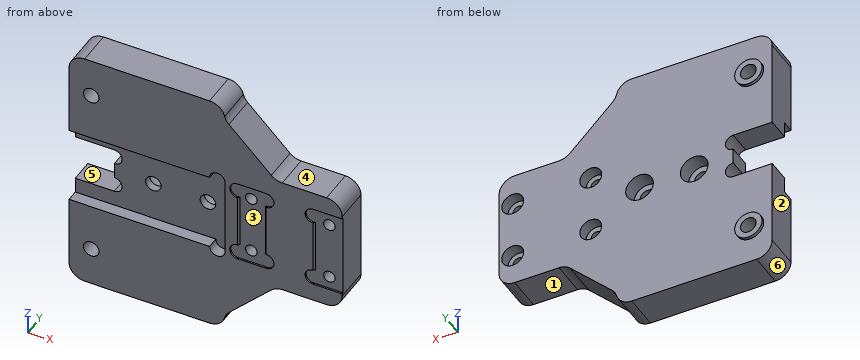
from build123d import *

# Parameters (mm, degrees)
SKETCH1_R               = 12
BOSS_EXTRUDE1_DEPTH     = 4.5
SKETCH2_R               = 1.7
CUT_EXTRUDE1_DEPTH      = 91.980767198
FILLET1_R               = 4
CUT_EXTRUDE4_DEPTH      = 91.980767198
FILLET3_R               = 4
SKETCH6_R               = 1.5
CUT_EXTRUDE5_DEPTH      = 41
CUT_EXTRUDE6_START      = -6
SKETCH7_W               = 30
SKETCH7_H               = 20
CUT_EXTRUDE6_DEPTH      = 3
SKETCH8_W               = 60
SKETCH8_H               = 17
CUT_EXTRUDE8_DEPTH      = 9
FILLET6_R               = 4
SKETCH9_W               = 40
SKETCH9_H               = 22.25
BOSS_EXTRUDE3_DEPTH     = 9
FILLET7_R               = 4
SKETCH13_R              = 3.5
BOSS_EXTRUDE5_DEPTH     = 0.8
CUT_EXTRUDE9_DEPTH      = 2
CUT_EXTRUDE9_DEPTH_BACK = 9
SKETCH10_R              = 2
BOSS_EXTRUDE4_DEPTH     = 9
SKETCH14_R              = 2
CUT_EXTRUDE10_DEPTH     = 16
SKETCH15_W              = 7.5
SKETCH15_H              = 21.7
CUT_EXTRUDE11_DEPTH     = 0.4
CHAMFER2_SIZE           = 0.4
CHAMFER3_SIZE           = 0.6
SKETCH16_W              = 4
SKETCH16_H              = 6
BOSS_EXTRUDE6_DEPTH     = 10
SKETCH17_R              = 2
CUT_EXTRUDE12_DEPTH     = 12.4
SKETCH18_R              = 3.55
CUT_EXTRUDE13_DEPTH     = 4
SKETCH19_R              = 2.8
CUT_EXTRUDE14_DEPTH     = 3
SKETCH20_R              = 2
CUT_EXTRUDE15_DEPTH     = 0.4
FILLET8_R               = 4
SKETCH21_R              = 2
CUT_EXTRUDE16_DEPTH     = 3


# Some blends are built 0.0001 mm under size
with BuildPart() as part:
    # Sketch1 → Boss-Extrude1 (new, symmetric)
    with BuildSketch(Plane(origin=(0, 0, 0), x_dir=(1, 0, 0), z_dir=(0, 1, 0))):
        Polygon((21.5, 20), (21.5, -20), (-20.5, -32.5), (-84.5, -32.5), (-84.5, 32.5), (-20.5, 32.5), align=None)
        with Locations(Location((0, 0, 0), (0, 0, 270))):
            Circle(SKETCH1_R, mode=Mode.SUBTRACT)
    extrude(amount=BOSS_EXTRUDE1_DEPTH, both=True)

    # Sketch2 → Cut-Extrude1 (cut, through all)
    with BuildSketch(Plane(origin=(0, 4.5, 0), x_dir=(1, 0, 0), z_dir=(0, 1, 0))):
        with Locations(Location((15.5, 15.5, 0), (0, 0, 270))):
            Circle(SKETCH2_R)
        with Locations(Location((-15.5, 15.5, 0), (0, 0, 270))):
            Circle(SKETCH2_R)
        with Locations(Location((-15.5, -15.5, 0), (0, 0, 270))):
            Circle(SKETCH2_R)
        with Locations(Location((15.5, -15.5, 0), (0, 0, 270))):
            Circle(SKETCH2_R)
        with Locations(Location((-19.5, 27.5, 0), (0, 0, 270))):
            Circle(SKETCH2_R)
        with Locations(Location((-19.5, -27.5, 0), (0, 0, 270))):
            Circle(SKETCH2_R)
    extrude(amount=-CUT_EXTRUDE1_DEPTH, mode=Mode.SUBTRACT)

    # Fillet1
    fillet1_edges = [part.edges().sort_by_distance(p)[0] for p in [
        (-20.5, 0, 32.5),
        (-84.5, 0, 32.5),
        (-84.5, 0, -32.5),
        (-20.5, 0, -32.5),
        (21.5, 0, -20),
        (21.5, 0, 20),
    ]]
    fillet(fillet1_edges, radius=FILLET1_R)

    # Sketch5 → Cut-Extrude4 (cut, through all)
    with BuildSketch(Plane(origin=(0, 4.5, 0), x_dir=(1, 0, 0), z_dir=(0, 1, 0))):
        Polygon((-24.5, 32.5), (-24.5, 10), (-24.5, -10), (-24.5, -32.5), (26.912022907, -32.5), (26.912022907, 32.5), align=None)
    extrude(amount=-CUT_EXTRUDE4_DEPTH, mode=Mode.SUBTRACT)

    # Fillet3
    fillet3_edges = [part.edges().sort_by_distance(p)[0] for p in [
        (-24.5, 0, -32.5),
        (-24.5, 0, 32.5),
    ]]
    fillet(fillet3_edges, radius=FILLET3_R)

    # Sketch6 → Cut-Extrude5 (cut)
    with BuildSketch(Plane.XZ.offset(4.5)):
        with Locations(Location((-47.999989197, -7.5, 0), (0, 0, 270))):
            Circle(SKETCH6_R)
        with Locations(Location((-47.999989197, 7.5, 0), (0, 0, 270))):
            Circle(SKETCH6_R)
        with Locations(Location((-27.999989197, 7.5, 0), (0, 0, 270))):
            Circle(SKETCH6_R)
        with Locations(Location((-27.999989197, -7.5, 0), (0, 0, 270))):
            Circle(SKETCH6_R)
    extrude(amount=-CUT_EXTRUDE5_DEPTH, mode=Mode.SUBTRACT)

    # Sketch7 → Cut-Extrude6 (cut)
    with BuildSketch(Plane(origin=(0, 4.5, 0), x_dir=(1, 0, 0), z_dir=(0, 1, 0)).offset(CUT_EXTRUDE6_START)):
        with Locations((-69.5, 0)):
            Rectangle(SKETCH7_W, SKETCH7_H)
    extrude(amount=-CUT_EXTRUDE6_DEPTH, mode=Mode.SUBTRACT)

    # Sketch8 → Cut-Extrude8 (cut)
    with BuildSketch(Plane(origin=(0, 4.5, 0), x_dir=(1, 0, 0), z_dir=(0, 1, 0))):
        with Locations((-54.5, 24)):
            Rectangle(SKETCH8_W, SKETCH8_H)
        with Locations((-54.5, -24)):
            Rectangle(SKETCH8_W, SKETCH8_H)
    extrude(amount=-CUT_EXTRUDE8_DEPTH, mode=Mode.SUBTRACT)

    # Fillet6
    fillet6_edges = [part.edges().sort_by_distance(p)[0] for p in [
        (-24.5, 0, -15.5),
        (-24.5, 0, 15.5),
    ]]
    fillet(fillet6_edges, radius=FILLET6_R)

    # Sketch9 → Boss-Extrude3 (add)
    with BuildSketch(Plane(origin=(0, 4.5, 0), x_dir=(1, 0, 0), z_dir=(0, 1, 0))):
        with Locations((-74.5, 21.125)):
            Rectangle(SKETCH9_W, SKETCH9_H)
        with Locations((-74.5, -21.125)):
            Rectangle(SKETCH9_W, SKETCH9_H)
    extrude(amount=-BOSS_EXTRUDE3_DEPTH)

    # Fillet7
    fillet7_edges = [part.edges().sort_by_distance(p)[0] for p in [
        (-54.5, 0, -32.25),
        (-94.5, 0, -32.25),
        (-54.5, 0, 32.25),
        (-94.5, 0, 32.25),
    ]]
    fillet(fillet7_edges, radius=FILLET7_R)

    # Sketch13 → Boss-Extrude5 (add)
    with BuildSketch(Plane(origin=(0, 4.5, 0), x_dir=(1, 0, 0), z_dir=(0, 1, 0))):
        with Locations(Location((-88.81, 22.25, 0), (0, 0, 90))):
            Circle(SKETCH13_R)
        with Locations(Location((-88.81, -22.25, 0), (0, 0, 90))):
            Circle(SKETCH13_R)
    extrude(amount=BOSS_EXTRUDE5_DEPTH)

    # Sketch10 → Cut-Extrude9 (cut, two sides: drawn at the far end of the back side and taken through both)
    with BuildSketch(Plane(origin=(0, 4.5, 0), x_dir=(1, 0, 0), z_dir=(0, 1, 0)).offset(-CUT_EXTRUDE9_DEPTH_BACK)):
        with Locations(Location((-88.81, -22.25, 0), (0, 0, 90))):
            Circle(SKETCH10_R)
        with Locations(Location((-88.81, 22.25, 0), (0, 0, 90))):
            Circle(SKETCH10_R)
    extrude(amount=CUT_EXTRUDE9_DEPTH + CUT_EXTRUDE9_DEPTH_BACK, mode=Mode.SUBTRACT)

    # Sketch11 → Boss-Extrude4 (add)
    with BuildSketch(Plane(origin=(0, 4.5, 0), x_dir=(1, 0, 0), z_dir=(0, 1, 0))):
        Polygon((-54.5, 28.25), (-41.5, 15.5), (-54.5, 15.5), align=None)
        Polygon((-54.5, -28.25), (-41.5, -15.5), (-54.5, -15.5), align=None)
    extrude(amount=-BOSS_EXTRUDE4_DEPTH)

    # Sketch14 → Cut-Extrude10 (cut)
    with BuildSketch(Plane.XZ.offset(1.5)):
        with Locations(Location((-74.5, 0, 0), (0, 0, 270))):
            Circle(SKETCH14_R)
        with Locations(Location((-60.5, 0, 0), (0, 0, 270))):
            Circle(SKETCH14_R)
    extrude(amount=-CUT_EXTRUDE10_DEPTH, mode=Mode.SUBTRACT)

    # Sketch15 → Cut-Extrude11 (cut)
    with BuildSketch(Plane.XZ.offset(4.5)):
        with Locations((-28.25, 0)):
            Rectangle(SKETCH15_W, SKETCH15_H)
        with Locations((-47.75, 0)):
            Rectangle(SKETCH15_W, SKETCH15_H)
    extrude(amount=-CUT_EXTRUDE11_DEPTH, mode=Mode.SUBTRACT)

    # Chamfer2
    chamfer2_edges = [part.edges().sort_by_distance(p)[0] for p in [
        (-32, -4.1, 0),
        (-44, -4.1, 0),
    ]]
    chamfer(chamfer2_edges, length=CHAMFER2_SIZE - 0.0001)  # a hair under: the kernel refuses the full size

    # Chamfer3
    # the kernel refuses this chamfer: 0.6 mm, written as the material it adds along each edge
    with BuildSketch(Plane(origin=(-51.5, -4.1, -12.393009793), x_dir=(-0.027495876610584506, -0.9996219169112968, 0), z_dir=(0, 0, 1))) as chamfer3_piece_1_section:
        Polygon((CHAMFER3_SIZE * 0.999621916911, CHAMFER3_SIZE * 0.0274958766106), (-CHAMFER3_SIZE * 0.0274958766106, CHAMFER3_SIZE * 0.999621916911), (0, 0), align=None)
    chamfer3_piece_1 = extrude(amount=24.786019586, mode=Mode.PRIVATE)
    chamfer3_piece_1 = split(chamfer3_piece_1, bisect_by=Plane(origin=(-51.281581799, -4.5, -11.621504896), z_dir=(0, 1, 0)), keep=Keep.TOP, mode=Mode.PRIVATE)
    add(chamfer3_piece_1)

    # Sketch16 → Boss-Extrude6 (add)
    with BuildSketch(Plane.ZY.offset(84.5)):
        with Locations((-8, 1.5)):
            Rectangle(SKETCH16_W, SKETCH16_H)
        with Locations((8, 1.5)):
            Rectangle(SKETCH16_W, SKETCH16_H)
    extrude(amount=BOSS_EXTRUDE6_DEPTH)

    # Sketch17 → Cut-Extrude12 (cut)
    with BuildSketch(Plane(origin=(0, 4.5, 0), x_dir=(1, 0, 0), z_dir=(0, 1, 0))):
        with Locations((-84.5, 4)):
            Circle(SKETCH17_R)
        with Locations((-84.5, -4)):
            Circle(SKETCH17_R)
    extrude(amount=-CUT_EXTRUDE12_DEPTH, mode=Mode.SUBTRACT)

    # Sketch18 → Cut-Extrude13 (cut)
    with BuildSketch(Plane(origin=(0, 4.5, 0), x_dir=(1, 0, 0), z_dir=(0, 1, 0))):
        with Locations(Location((-74.5, 0, 0), (0, 0, 270))):
            Circle(SKETCH18_R)
        with Locations(Location((-60.5, 0, 0), (0, 0, 270))):
            Circle(SKETCH18_R)
    extrude(amount=-CUT_EXTRUDE13_DEPTH, mode=Mode.SUBTRACT)

    # Sketch19 → Cut-Extrude14 (cut)
    with BuildSketch(Plane(origin=(0, 4.5, 0), x_dir=(1, 0, 0), z_dir=(0, 1, 0))):
        with Locations(Location((-47.999989197, 7.5, 0), (0, 0, 270))):
            Circle(SKETCH19_R)
        with Locations(Location((-27.999989197, 7.5, 0), (0, 0, 270))):
            Circle(SKETCH19_R)
        with Locations(Location((-47.999989197, -7.5, 0), (0, 0, 270))):
            Circle(SKETCH19_R)
        with Locations(Location((-27.999989197, -7.5, 0), (0, 0, 270))):
            Circle(SKETCH19_R)
    extrude(amount=-CUT_EXTRUDE14_DEPTH, mode=Mode.SUBTRACT)

    # Sketch20 → Cut-Extrude15 (cut)
    with BuildSketch(Plane.XZ.offset(4.5)):
        with Locations((-32, 8.85)):
            Circle(SKETCH20_R)
        with Locations((-32, -8.85)):
            Circle(SKETCH20_R)
        with BuildLine():
            Line((-51.3, -6.85), (-50.9, -6.85))
            Line((-50.9, -6.85), (-50.9, -10.85))
            Line((-50.9, -10.85), (-51.3, -10.85))
            ThreePointArc((-51.3, -10.85), (-53.3, -8.85), (-51.3, -6.85))
        make_face()
        with BuildLine():
            Line((-44, -6.85), (-44.4, -6.85))
            Line((-44.4, -6.85), (-44.4, -10.85))
            Line((-44.4, -10.85), (-44, -10.85))
            ThreePointArc((-44, -10.85), (-42, -8.85), (-44, -6.85))
        make_face()
        with BuildLine():
            Line((-51.3, 6.85), (-50.9, 6.85))
            Line((-50.9, 6.85), (-50.9, 10.85))
            Line((-50.9, 10.85), (-51.3, 10.85))
            ThreePointArc((-51.3, 10.85), (-53.3, 8.85), (-51.3, 6.85))
        make_face()
        with BuildLine():
            Line((-44, 6.85), (-44.4, 6.85))
            Line((-44.4, 6.85), (-44.4, 10.85))
            Line((-44.4, 10.85), (-44, 10.85))
            ThreePointArc((-44, 10.85), (-42, 8.85), (-44, 6.85))
        make_face()
    extrude(amount=-CUT_EXTRUDE15_DEPTH, mode=Mode.SUBTRACT)

    # Fillet8
    fillet8_edges = [part.edges().sort_by_distance(p)[0] for p in [
        (-54.5, 0, -28.25),
        (-54.5, 0, 28.25),
        (-41.5, 0, -15.5),
        (-41.5, 0, 15.5),
    ]]
    fillet(fillet8_edges, radius=FILLET8_R)

    # Sketch21 → Cut-Extrude16 (cut)
    with BuildSketch(Plane.XZ.offset(4.5)):
        with Locations((-56.5, 10)):
            Circle(SKETCH21_R)
        with Locations((-56.5, -10)):
            Circle(SKETCH21_R)
    extrude(amount=-CUT_EXTRUDE16_DEPTH, mode=Mode.SUBTRACT)


solid = part.part
Model file for the job. Use its own axes, mm. Face numbers are marked on the shaded views. A direction names the side the tool comes from. Give positions to 0.01 mm unless a question says otherwise; leave off trailing zeros. Order: outer loops, then holes, each group sorted by start corner. A loop starts at its lowest first (then second) coordinate and runs counter-clockwise, first axis right, second up. Notation, with made-up numbers: (77.25, 1.25) - (86.25, 1.25) arc R30 cw to (86.25, 27.25) - close; hole circle Ø7 at (-12.5, 29.25). An arc over 180 degrees is marked (long way). Return JSON: item names as keys, results as strings.
1) Flat gauge pins, fed straight in: P1, Ø2, axis at x = -75.5, z = -0.5, coming from the +Y side; P2, Ø6, axis at x = -46.5, z = -7, coming from the +Y side; P3, Ø4, axis at x = -79.5, z = 6.5, coming from the -Y side. Where does each tip first touch, or does it go through?
Geometry says:
{"P1": "y = 0.5", "P2": "y = 4.5", "P3": "y = -1.5"}
2) Pull direction Z, two halves, no side cores. Call the marked faces 1, 2, 3 and 4: pulls with the +Z half, pulls with the -Z half, needs draft (parallel to the pull), parting line crosses it, or undercut.
Geometry says:
{"face 1": "pulls with the -Z half", "face 2": "needs draft", "face 3": "undercut", "face 4": "pulls with the +Z half"}
3) Probe line 1 (Z direction, x = -32, y = -4.3); line 2 (X direction, y = -1.45, z = -7.5); line 3 (X direction, y = 2.3, z = -7.5). List the from-to ranges inside material, lowest first. Write a range as from..to.
Geometry says:
{"line 1": "-15.5..-10.85, -6.85..6.85, 10.85..15.5", "line 2": "-94.5..-49.5, -46.5..-29.5, -26.5..-24.5", "line 3": "-94.5..-50.8, -45.2..-30.8, -25.2..-24.5"}
4) 3-axis set-ups, long thin cutter, end or side, ignore diameter. For the marked faces 5 and 6: which of +Z, -Z, +X, -X, +Y, -Y reach the whole face in a straight line?
Geometry says:
{"face 5": "-X, +Y, -Y", "face 6": "-Z, -X, +Y, -Y"}
5) Cut at B-B, the plane z = 0. Count the separate pieces of the cut face and the enclosed holes in it, plus the area to 3 significant figures.
Geometry says:
{"separate pieces": "3", "enclosed holes": "0", "area": "372 mm²"}
6) Cut at D-D, the plane z = 22.25. Give the cut face in (x, y), plus the area to 3 significant figures.
Geometry says:
{"outline": "(-94.5, -4.5) - (-90.81, -4.5) - (-90.81, 5.3) - (-92.31, 5.3) - (-92.31, 4.5) - (-94.5, 4.5) - close; (-86.81, -4.5) - (-48.38, -4.5) - (-48.38, 4.5) - (-85.31, 4.5) - (-85.31, 5.3) - (-86.81, 5.3) - close", "area": "381 mm²"}
7) Cut at C-C, the plane x = -60.5. Give the cut face in (y, z).
Geometry says:
{"outline": "(-4.5, -32.25) - (4.5, -32.25) - (4.5, -3.55) - (0.5, -3.55) - (0.5, -2) - (-1.5, -2) - (-1.5, -10) - (-4.5, -10) - close; (-4.5, 10) - (-1.5, 10) - (-1.5, 2) - (0.5, 2) - (0.5, 3.55) - (4.5, 3.55) - (4.5, 32.25) - (-4.5, 32.25) - close"}
8) Cut at A-A, the plane x = -88.81. Give the cut face in (y, z), plus the area to 3 significant figures.
Geometry says:
{"outline": "(-4.5, -32.25) - (4.5, -32.25) - (4.5, -25.75) - (5.3, -25.75) - (5.3, -24.25) - (-4.5, -24.25) - close; (-4.5, -20.25) - (5.3, -20.25) - (5.3, -18.75) - (4.5, -18.75) - (4.5, -6) - (-1.5, -6) - (-1.5, -10) - (-4.5, -10) - close; (-4.5, 10) - (-1.5, 10) - (-1.5, 6) - (4.5, 6) - (4.5, 18.75) - (5.3, 18.75) - (5.3, 20.25) - (-4.5, 20.25) - close; (-4.5, 24.25) - (5.3, 24.25) - (5.3, 25.75) - (4.5, 25.75) - (4.5, 32.25) - (-4.5, 32.25) - close", "area": "381 mm²"}
